Model file for the job. Use its own axes, mm. A direction names the side the tool comes from. Round coordinates to 2 decimals unless told otherwise and drop trailing zeros. Order: outer loops, then holes, each group sorted by start corner. A loop starts at its lowest first (then second) coordinate and runs counter-clockwise, first axis right, second up. Notation, with made-up numbers: (16, -40) - (42, -40) arc R10 cw to (42, -26) - close; hole circle Ø1 at (17, 11.25). An arc over 180 degrees is marked (long way). Write item = value, one per line.
```python
from build123d import *

# Parameters (mm, degrees)
SKETCH_1_R      = 10
SKETCH_1_R_2    = 1.5
EXTRUDE_1_DEPTH = 3
EXTRUDE_2_DEPTH = 13


with BuildPart() as part:
    # 草图1 → 凸台-拉伸1 (new body)
    with BuildSketch(Plane(origin=(0, 0, 0), x_dir=(1, 0, 0), z_dir=(0, 1, 0))):
        with Locations(Location((0, 0, 0), (0, 0, 270))):
            Circle(SKETCH_1_R)
        with Locations(Location((0, 6.5, 0), (0, 0, 270))):
            Circle(SKETCH_1_R_2, mode=Mode.SUBTRACT)
        with Locations(Location((5.629165125, -3.25, 0), (0, 0, 270))):
            Circle(SKETCH_1_R_2, mode=Mode.SUBTRACT)
        with Locations(Location((-5.629165125, -3.25, 0), (0, 0, 270))):
            Circle(SKETCH_1_R_2, mode=Mode.SUBTRACT)
    extrude(amount=EXTRUDE_1_DEPTH)

    # 草图2 → 凸台-拉伸2 (add)
    with BuildSketch(Plane(origin=(0, 0, 0), x_dir=(1, 0, 0), z_dir=(0, 1, 0))):
        with BuildLine():
            Line((-1.05, 1), (1.05, 1))
            ThreePointArc((1.05, 1), (0, -1.45), (-1.05, 1))
        make_face()
    extrude(amount=EXTRUDE_2_DEPTH)


solid = part.part
```
1) Wall check: line 1 along X through (y, z) = (1.3, 3.25); line 2 along Y through (x, z) = (5.25, 5.75); line 3 along Z through (x, y) = (-6.25, 1.25). Give the ranges that are in metal, low to high.
Conclusion:
line_1 = -9.46 to -7.13, -4.13 to 4.13, 7.13 to 9.46
line_2 = 0 to 3
line_3 = -7.81 to 1.88, 4.62 to 7.81
2) Mould opens along X. For faces 3 (the face through (0, 0, 0)), 4 (the face through (0.05, 7.93, 1.45)), 5 (the face through (4.298, 1.479, 3.942)) say: +X half, -X half, draft (parallel to the pull), parting line (faces both ways), or undercut.
Conclusion:
face_3 = draft
face_4 = parting line
face_5 = undercut
3) Cut at C-C (z = 0). Write the cut outline in (x, y), and give its area (3 significant figures).
Conclusion:
outline = (-10, 0) - (10, 0) - (10, 3) - (1.45, 3) - (1.45, 13) - (-1.45, 13) - (-1.45, 3) - (-10, 3) - close
area = 89.0 mm^2
4) Cut at D-D (z = 4). Write the cut outline in (x, y), and give its area (3 significant figures).
Conclusion:
outline = (-9.17, 0) - (-6.93, 0) - (-6.93, 3) - (-9.17, 3) - close; (-4.33, 0) - (4.33, 0) - (4.33, 3) - (-4.33, 3) - close; (6.93, 0) - (9.17, 0) - (9.17, 3) - (6.93, 3) - close
area = 39.4 mm^2
5) Cut at B-B (x = -6). Write the cut outline in (y, z), and give its area (3 significant figures).
Conclusion:
outline = (0, -8) - (3, -8) - (3, 1.8) - (0, 1.8) - close; (0, 4.7) - (3, 4.7) - (3, 8) - (0, 8) - close
area = 39.3 mm^2
6) Flat gauge pins, fed straight in: pin 1 Ø4 at (x, z) = (5.63, 3.25) entering from -Y; pin 2 Ø1.7 at (x, y) = (0, 9.5) entering from -Z; pin 3 Ø4 at (x, z) = (0, -6.5) entering from +Y; pin 4 Ø2 at (y, z) = (11.5, -1) entering from +X. Where does each tip first touch, or does it go through?
Conclusion:
pin_1 = 0
pin_2 = -1
pin_3 = 3
pin_4 = 1.45
7) Cut at A-A (z = -5.75). Write the cut outline in (x, y), and give its area (3 significant figures).
Conclusion:
outline = (-8.18, 0) - (-1.3, 0) - (-1.3, 3) - (-8.18, 3) - close; (1.3, 0) - (8.18, 0) - (8.18, 3) - (1.3, 3) - close
area = 41.3 mm^2
8) 3-axis set-ups, long thin cutter, end or side, ignore diameter. For faces 1 (the face through (0, 8, -1)), 2 (the face through (-9.76, 1.48, -2.17)): which of +Z, -Z, +X, -X, +Y, -Y reach the whole face in a straight line?
Conclusion:
face_1 = -Z, +X, -X, +Y
face_2 = +Y, -Y
